For this review, take the finished solid that the model builds, in its own axes (mm). Coordinates: 2 decimals unless noted, no trailing zeros. Write each loop counter-clockwise with the first axis right and the second up, starting at its lowest first coordinate (ties: lowest second). Pieces come first, ordered by that corner, then holes. Notation, with made-up numbers: M 9,77.5 L 43,77.5 A7 cw 43,88.5 Z; hole C -9,30 d2. An arc over 180 degrees is marked long. One line per question, with ' | ' between items.
Autodesk Inventor part; units mm, degrees
ref_plane "YZ Plane" through (0, 0, 0) normal (1, 0, 0) x (0, 1, 0)
ref_plane "XZ Plane" through (0, 0, 0) normal (0, 1, 0) x (-1, 0, 0)
ref_plane "XY Plane" through (0, 0, 0) normal (0, 0, 1) x (1, 0, 0)
sketch "Sketch2" plane through (0, 0, 0) normal (0, 1, 0) x (-1, 0, 0)
  circle A0 centre (0, 0) radius 29
  circle A1 centre (0, 0) radius 28
  dimension "d14" = 58
  dimension "d15" = 56
extrude "Extrusion2" add sketch "Sketch2" along normal blind 158
fillet "Fillet1" radius 2 1 edges at (29, 0, 0)
fillet "Fillet2" radius 2 1 edges at (29, 158, 0)
properties part number "snow_can_middle"
1. Take a section at B-B on x = 0. State the section outline as (y, z) points, plus the area to 3 significant figures.
Computed values:
outline: M 0,-28 A2 ccw 1.73,-29 L 156.27,-29 A2 ccw 158,-28 Z; M 0,28 L 158,28 A2 ccw 156.27,29 L 1.73,29 A2 ccw Z | area: 314 mm2
2. Take a section at A-A on z = 0. State the section outline as (x, y) points, plus the area to 3 significant figures.
Computed values:
outline: M -29,1.73 A2 ccw -28,0 L -28,158 A2 ccw -29,156.27 Z; M 28,0 A2 ccw 29,1.73 L 29,156.27 A2 ccw 28,158 Z | area: 314 mm2
3. Take a section at C-C on y = 102.5. State the section outline as (x, z) points, plus the area to 3 significant figures.
Computed values:
outline: C 0,0 d58; hole C 0,0 d56 | area: 179 mm2
4. For line 1 along Z through (x, y) = (0, 124.5); line 2 along Z through (x, y) = (-5, 114.5); line 3 along X through (y, z) = (70, 21.5), list the stretches that pass through material, from the lowest coordinate up.
Computed values:
line 1: z = -29 to -28, 28 to 29 | line 2: z = -28.57 to -27.55, 27.55 to 28.57 | line 3: x = -19.46 to -17.94, 17.94 to 19.46
5. Draft analysis for pull direction Z (two halves, no side actions). For faces 1 (the cylindrical face through (-13.38, 77.92, 25.73)), 2 (the cylindrical face through (-25.865, 77.894, 10.724)), state which applies: pulls with the +Z half, pulls with the -Z half, needs draft (parallel to the pull), parting line crosses it, or undercut.
Computed values:
face 1: parting line crosses it | face 2: undercut
6. Clearance check with flat-ended pins moving along their axes: P1, Ø1.5, axis at x = 13, y = 28.5, coming from the -Z side; P2, Ø6, axis at x = -18, y = 140.5, coming from the -Z side; P3, Ø3, axis at x = -3, y = 67.5, coming from the +Z side. State where each tip first meets the part, or that it passes through.
Computed values:
P1: stops at z = -26.29 | P2: stops at z = -24.82 | P3: stops at z = 28.96
